Work out the finished part from the listing and answer in its coordinate system (mm). A direction names the side the tool comes from. Give positions to 0.01 mm unless a question says otherwise; leave off trailing zeros. Order: outer loops, then holes, each group sorted by start corner. A loop starts at its lowest first (then second) coordinate and runs counter-clockwise, first axis right, second up. Notation, with made-up numbers: (78, 14) - (136, 14) arc R32 cw to (136, 50) - close; hole circle Ø7 at (28.5, 6). An arc over 180 degrees is marked (long way). Write each question's results on one line, items separated by ' | '.
from build123d import *

# Parameters (mm, degrees)
EXTRUDE_1_DEPTH     = 15
SKETCH_2_W          = 72.5
SKETCH_2_H          = 52
CUT_EXTRUDE_1_DEPTH = 8
SKETCH_3_W          = 72.5
SKETCH_3_H          = 8
CUT_EXTRUDE_4_DEPTH = 12.5


with BuildPart() as part:
    # Sketch 1 → Extrude 1 (new body)
    with BuildSketch(Plane.XY):
        with BuildLine():
            Line((0, 0), (19.671242882, 0))
            Line((19.671242882, 0), (31.588778808, 10))
            Line((31.588778808, 10), (200, 10))
            Line((200, 10), (200, -55.775476447))
            Line((200, -55.775476447), (195.298724865, -55.775476447))
            Line((195.298724865, -55.775476447), (164.192027956, -61.260426393))
            ThreePointArc((164.192027956, -61.260426393), (152.722113491, -58.588242921), (142.85786008, -65.0222158))
            Line((142.85786008, -65.0222158), (120.298724865, -69))
            Line((120.298724865, -69), (100.298724865, -69))
            ThreePointArc((100.298724865, -69), (95.026646927, -81.727922061), (82.298724865, -87))
            Line((82.298724865, -87), (67.298724865, -87))
            ThreePointArc((67.298724865, -87), (54.570802804, -81.727922061), (49.298724865, -69))
            Line((49.298724865, -69), (36.111333122, -69))
            Line((36.111333122, -69), (19.298724865, -52.187391743))
            Line((19.298724865, -52.187391743), (19.298724865, -30))
            Line((19.298724865, -30), (0, -30))
            Line((0, -30), (0, 0))
        make_face()
        with BuildLine():
            Line((67.298724865, -53), (82.298724865, -53))
            ThreePointArc((82.298724865, -53), (98.298724865, -69), (82.298724865, -85))
            Line((82.298724865, -85), (67.298724865, -85))
            ThreePointArc((67.298724865, -85), (51.298724865, -69), (67.298724865, -53))
        make_face(mode=Mode.SUBTRACT)
    extrude(amount=EXTRUDE_1_DEPTH)

    # Sketch 2 → Cut-Extrude 1 (cut)
    with BuildSketch(Plane.XY.offset(15)):
        with Locations((74.798724865, -24)):
            Rectangle(SKETCH_2_W, SKETCH_2_H)
    extrude(amount=-CUT_EXTRUDE_1_DEPTH, mode=Mode.SUBTRACT)

    # Sketch 3 → Cut-Extrude 4 (cut)
    with BuildSketch(Plane.XY.offset(15)):
        with Locations((74.798724865, 6)):
            Rectangle(SKETCH_3_W, SKETCH_3_H)
    extrude(amount=-CUT_EXTRUDE_4_DEPTH, mode=Mode.SUBTRACT)


solid = part.part
1. A cutting plane is placed at B-B, the plane x = 63. Write down the section's boundary in (y, z).
Answer list:
outline: (-86.48, 0) - (-84.41, 0) - (-84.41, 15) - (-86.48, 15) - close; (-53.59, 0) - (10, 0) - (10, 2.5) - (2, 2.5) - (2, 7) - (-50, 7) - (-50, 15) - (-53.59, 15) - close
2. A tool of negligible diameter and unlimited length cuts with its end or side. For faces 1 (the face through (10, 0, 7)), 2 (the face through (74, -24, 7)), 3 (the face through (75, -85, 7)), from which of +Z, -Z, +X, -X, +Y, -Y can it reach the whole face along a straight path? Write none if from no direction.
Answer list:
face 1: +Z, -Z, -X, +Y | face 2: +Z, +Y | face 3: +Z, -Z
3. A cutting plane is placed at A-A, the plane z = 10.5. Write down the section's boundary in (x, y).
Answer list:
outline: (0, -30) - (19.3, -30) - (19.3, -52.19) - (36.11, -69) - (49.3, -69) arc R18 ccw to (67.3, -87) - (82.3, -87) arc R18 ccw to (100.3, -69) - (120.3, -69) - (142.86, -65.02) arc R15 cw to (164.19, -61.26) - (195.3, -55.78) - (200, -55.78) - (200, 10) - (111.05, 10) - (111.05, -50) - (38.55, -50) - (38.55, 10) - (31.59, 10) - (19.67, 0) - (0, 0) - close; hole (67.3, -85) - (82.3, -85) arc R16 ccw to (82.3, -53) - (67.3, -53) arc R16 ccw to start
4. Given P1, Ø4, axis at x = 43, z = 7.5, coming from the +Y side; P2, Ø4, axis at x = 196.5, z = 9.5, coming from the -Y side; P3, Ø6, axis at y = -48, z = 7.5, coming from the -X side, each flat-ended and moving along its own axis, determine where each tip first touches the part or whether it passes through.
Answer list:
P1: y = 2 | P2: y = -55.92 | P3: x = 19.3
5. A cutting plane is placed at C-C, the plane y = -11.5. Write down the section's boundary in (x, z).
Answer list:
outline: (0, 0) - (200, 0) - (200, 15) - (111.05, 15) - (111.05, 7) - (38.55, 7) - (38.55, 15) - (0, 15) - close
6. A cutting plane is placed at D-D, the plane y = -74.5. Write down the section's boundary in (x, z).
Answer list:
outline: (50.16, 0) - (52.27, 0) - (52.27, 15) - (50.16, 15) - close; (97.32, 0) - (99.44, 0) - (99.44, 15) - (97.32, 15) - close
7. Determine the mould class of faces 4 (the face through (95.166, -81.587, 7.395)), 5 (the face through (124, -27, 15)), 6 (the face through (51.303, -69.352, 7.395)) for opening direction Y: +Y half, -Y half, draft (parallel to the pull), parting line (faces both ways), or undercut.
Answer list:
face 4: -Y half | face 5: draft | face 6: undercut
8. Straight lines are drawn through the part: line 1 (X direction, y = -31.5, z = 14.5); line 2 (X direction, y = -14, z = 14); line 3 (Y direction, x = 48.5, z = 1.5). For each, find the intervals that lie inside material, in ascending order. Write a range as [from, to].
Answer list:
line 1: [19.3, 38.55], [111.05, 200] | line 2: [0, 38.55], [111.05, 200] | line 3: [-69, 10]
